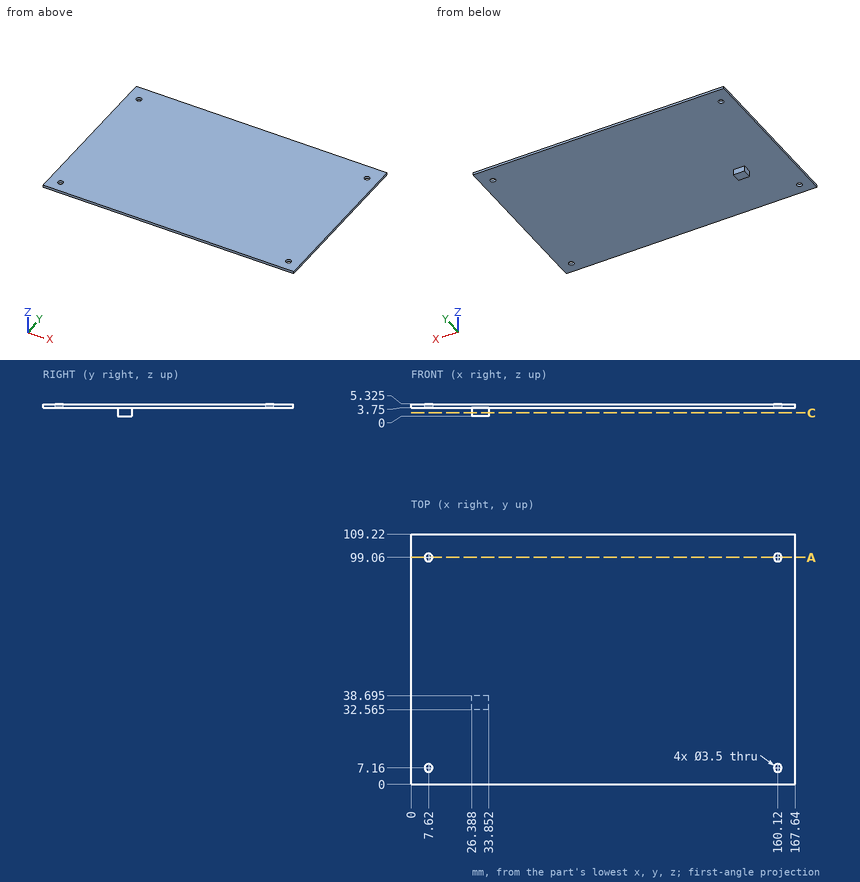
Geometry check sheet. Reference: drawing and pictorial views, mm from the part's lowest x, y, z. Coordinates: 2 decimals unless noted, no trailing zeros. Order: outer loops, then holes, each group sorted by start corner. A loop starts at its lowest first (then second) coordinate and runs counter-clockwise, first axis right, second up. Notation, with made-up numbers: (60, 17) -> (87, 17) arc R22 ccw to (87, 52) -> close; hole circle Ø8 at (28, 86). An arc over 180 degrees is marked (long way). Put each result on its own line as item: value. Start each with the question number.
1) Cross-section at A-A (y = 99.06). State how many separate pieces and enclosed holes the cut face has, plus the area to 3 significant figures.
2) Cross-section at C-C (z = 1.4). Enter the section's corners in (x, y) (1 decimal).
3) Material ranges on L1, parallel to Y at x = 7.62, z = 4.3; L2, parallel to X at y = 99.06, z = 4.5; L3, parallel to Y at x = 30, z = 0.45 (1 decimal), recorded low to high.
4) Go/stop test with flat-tipped pins: pin 1 (10 mm diameter, centred on x = 31, y = 23, fed in from -Z); pin 2 (1.9 mm diameter, centred on x = 30, z = 2.5, fed in from -Y) (1 decimal); pin 3 (1.9 mm diameter, centred on x = 32, z = 1.5, fed in from +Y) (1 decimal); pin 4 (3 mm diameter, centred on x = 160.12, y = 7.16, fed in from +Z). Record where each tip stops, or that it passes through.
Geometry check:
1. separate pieces: 3
1. enclosed holes: 0
1. area: 253 mm^2
2. outline: (26.4, 32.6) -> (33.9, 32.6) -> (33.9, 38.7) -> (26.4, 38.7) -> close
3. L1: y = 0 to 5.41, 8.91 to 97.31, 100.81 to 109.22
3. L2: x = 0 to 5.87, 9.37 to 158.37, 161.87 to 167.64
3. L3: y = 32.6 to 38.7
4. pin 1: stops at z = 3.75
4. pin 2: stops at y = 32.6
4. pin 3: stops at y = 38.7
4. pin 4: passes through
